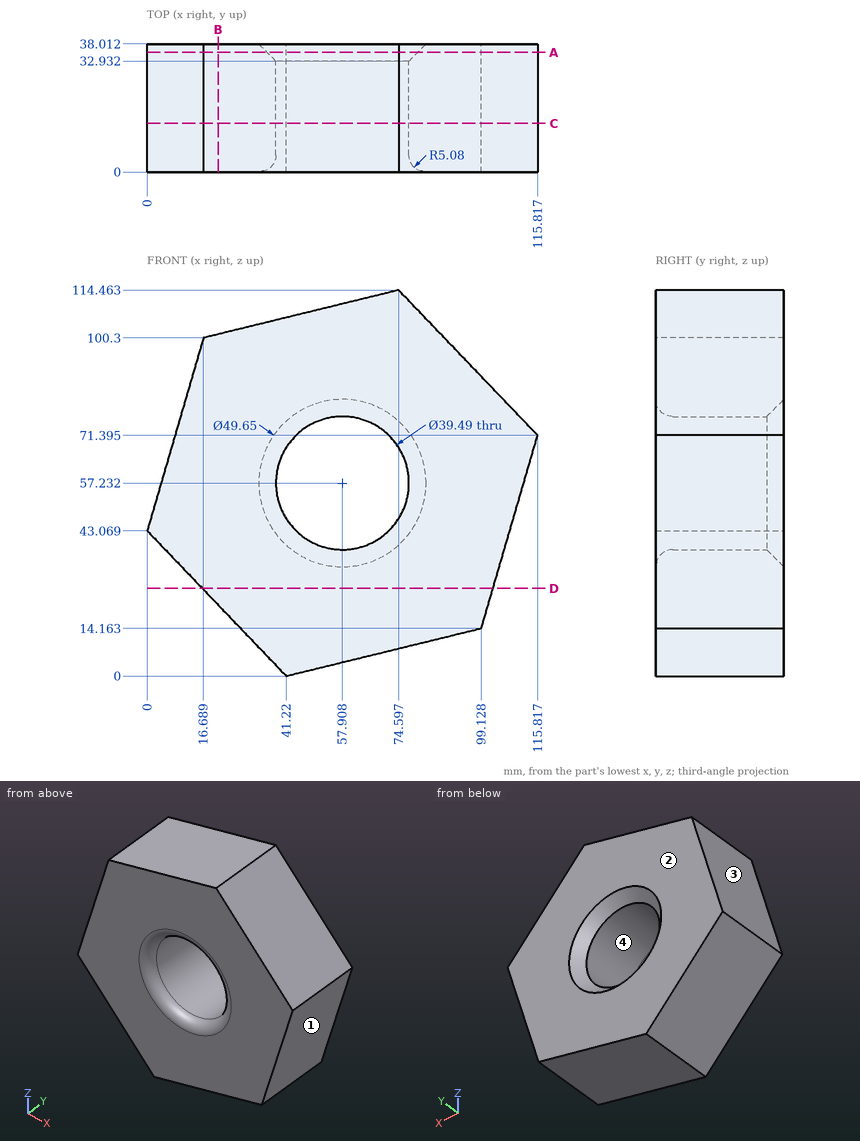
The drawing under review shows one solid part. Ordinate dimensions are in mm from its lowest x, y, z. Coordinates: 2 decimals unless noted, no trailing zeros. Order: outer loops, then holes, each group sorted by start corner. A loop starts at its lowest first (then second) coordinate and runs counter-clockwise, first axis right, second up. Notation, with made-up numbers: M -9,5 L 43,5 A20 ccw 43,33 Z; hole C -8.75,57 d8. An arc over 180 degrees is marked long. Use a Markdown table: item, result.
(1) Add section C-C (y = 14.5). Give the boundary of the cut face in (x, z) (1 decimal).
Worked answers:
| item | result |
|---|---|
| outline | M 0,43.1 L 41.2,0 L 99.1,14.2 L 115.8,71.4 L 74.6,114.5 L 16.7,100.3 Z; hole C 57.9,57.2 d39.5 |
(2) Add section B-B (x = 21). Give the boundary of the cut face in (y, z) (1 decimal), then the cut area to 3 significant figures.
Worked answers:
| item | result |
|---|---|
| outline | M 0,21.1 L 38,21.1 L 38,101.4 L 0,101.4 Z |
| area | 3,050 mm2 |
(3) Wall thickness on probe 1 along X at (y, z) = (28, 51) (1 decimal); probe 2 along X at (y, z) = (19.5, 44) (1 decimal); probe 3 along Z at (x, y) = (42, 12.5) (1 decimal): over which ranges is each line inside the solid? List them lowest first.
Worked answers:
| item | result |
|---|---|
| probe 1 | x = 2.3 to 39.2, 76.6 to 109.9 |
| probe 2 | x = 0.3 to 43.3, 72.6 to 107.8 |
| probe 3 | z = 0.2 to 45.5, 68.9 to 106.5 |
(4) Add section A-A (y = 35.5). Give the boundary of the cut face in (x, z) (1 decimal), then the cut area to 3 significant figures.
Worked answers:
| item | result |
|---|---|
| outline | M 0,43.1 L 41.2,0 L 99.1,14.2 L 115.8,71.4 L 74.6,114.5 L 16.7,100.3 Z; hole C 57.9,57.2 d44.6 |
| area | 7,670 mm2 |
(5) For P1, Ø4, axis at x = 25.5, z = 14.5, coming from the -Y side; P2, Ø1, axis at y = 19.5, z = 26, coming from the +X side (1 decimal); P3, Ø10, axis at y = 8.5, z = 50.5, coming from the -X side; P4, Ø4, axis at y = 26, z = 78.5, coming from the +X side, all flat-tipped, find the tip position at first contact; note any pin that passes through.
Worked answers:
| item | result |
|---|---|
| P1 | stops at y = 0 |
| P2 | stops at x = 102.7 |
| P3 | stops at x = 0.71 |
| P4 | stops at x = 110.93 |
(6) Draft analysis for pull direction X (two halves, no side actions). For the marked faces 1, 2, 3 and 4, state which applies: released by +X, released by -X, zero draft, split by the parting line, or undercut.
Worked answers:
| item | result |
|---|---|
| face 1 | released by +X |
| face 2 | zero draft |
| face 3 | released by -X |
| face 4 | undercut |
(7) Add section D-D (z = 26). Give the boundary of the cut face in (x, y) (1 decimal).
Worked answers:
| item | result |
|---|---|
| outline | M 16.3,0 L 102.6,0 L 102.6,38 L 16.3,38 Z |
